Build history of the part. All positions in model axes, mm. Face numbers are marked on the shaded views. Give positions to 0.01 mm unless a question says otherwise; leave off trailing zeros. Order: outer loops, then holes, each group sorted by start corner. A loop starts at its lowest first (then second) coordinate and runs counter-clockwise, first axis right, second up. Notation, with made-up numbers: (43, -1) - (59, -1) arc R23 ccw to (59, 35) - close; hole circle Ø11 at (65.25, 61.25). An arc over 180 degrees is marked (long way). Write each question's results on one line, items separated by ' | '. Start each with the question number.
1) Drop flat-ended pins along their axis: pin 1 Ø2 at (x, y) = (-3.5, -59) entering from +Z; pin 2 Ø3 at (x, y) = (0, 8) entering from -Z; pin 3 Ø2 at (x, z) = (-9.5, 2.5) entering from -Y; pin 4 Ø1.5 at (x, z) = (-7, 3.5) entering from -Y. Give the stop position or say it passes through.
2) Two-plate mould, pull along X, no slides. Class the marked faces 1, 2, 3 and 4: +X half, -X half, draft (parallel to the pull), parting line (faces both ways), or undercut.
3) Cut at B-B on z = 2. List the corners of the cut face in (x, y).
4) Cut at D-D on x = 8. List the corners of the cut face in (y, z), plus the area to 3 significant figures.
5) Cut at A-A on x = 0. List the corners of the cut face in (y, z), plus the area to 3 significant figures.
6) Cut at C-C on y = -8. List the corners of the cut face in (x, z).
7) Drill centre lines: line 1 along X through (y, z) = (0, 4.6); line 2 along Y through (x, z) = (0, 4.5); line 3 along Z through (x, y) = (8.5, -7.5). Where is each one in solid material? Low to high. Write a range as from..to.
from build123d import *

# Parameters (mm, degrees)
ESQUISSE1_R             = 15
ESQUISSE1_R_2           = 1.8
ESQUISSE1_R_3           = 4
BOSS_EXTRU_1_DEPTH      = 7
CONG_1_R                = 1.5
CONG_2_R                = 6
ESQUISSE3_R             = 12
ENL_V_MAT_EXTRU_2_DEPTH = 3.5


with BuildPart() as part:
    # Esquisse1 → Boss.-Extru.1 (new body)
    # profile 1 of 2: a face of its own
    with BuildSketch(Plane.XY):
        with BuildLine():
            ThreePointArc((15, 0), (0, -15), (-15, 0))
            Line((-15, 0), (-15, -80))
            Line((-15, -80), (15, -20))
            Line((15, -20), (15, 0))
        make_face()
    # profile 2 of 2: a face of its own
    with BuildSketch(Plane.XY):
        Circle(ESQUISSE1_R)
        with Locations((-8, 0)):
            Circle(ESQUISSE1_R_2, mode=Mode.SUBTRACT)
        with Locations((0, -8)):
            Circle(ESQUISSE1_R_2, mode=Mode.SUBTRACT)
        with Locations((8, 0)):
            Circle(ESQUISSE1_R_2, mode=Mode.SUBTRACT)
        with Locations((0, 8)):
            Circle(ESQUISSE1_R_2, mode=Mode.SUBTRACT)
        Circle(ESQUISSE1_R_3, mode=Mode.SUBTRACT)
    extrude(amount=BOSS_EXTRU_1_DEPTH)

    # Congé1
    cong_1_edges = [part.edges().sort_by_distance(p)[0] for p in [
        (-15, -80, 3.5),
    ]]
    fillet(cong_1_edges, radius=CONG_1_R)

    # Congé2
    cong_2_edges = [part.edges().sort_by_distance(p)[0] for p in [
        (15, -20, 3.5),
    ]]
    fillet(cong_2_edges, radius=CONG_2_R)

    # Esquisse3 → Enlèv. mat.-Extru.2 (cut)
    with BuildSketch(Plane(origin=(0, 0, 0), x_dir=(-1, 0, 0), z_dir=(0, 0, -1))):
        Circle(ESQUISSE3_R)
    extrude(amount=-ENL_V_MAT_EXTRU_2_DEPTH, mode=Mode.SUBTRACT)


solid = part.part
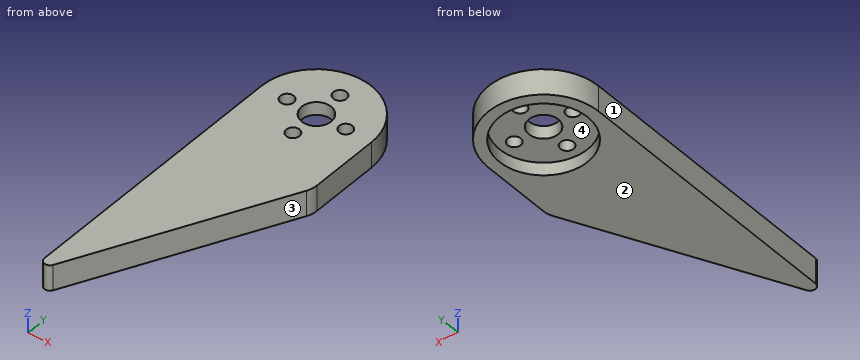
Results:
1) pin 1: z = 7 | pin 2: through | pin 3: y = -71 | pin 4: y = -65.5
2) face 1: -X half | face 2: draft | face 3: +X half | face 4: undercut
3) outline: (-15, -73.65) arc R1.5 ccw to (-12.16, -74.32) - (14.37, -21.27) arc R6 ccw to (15, -18.58) - (15, 0) arc R15 ccw to (-15, 0) - close; hole circle Ø24 at (0, 0)
4) outline: (-34, 0) - (-8.94, 0) - (-8.94, 3.5) - (-1.8, 3.5) - (-1.8, 7) - (-34, 7) - close; (1.8, 3.5) - (8.94, 3.5) - (8.94, 0) - (12.69, 0) - (12.69, 7) - (1.8, 7) - close | area: 252 mm^2
5) outline: (-50, 0) - (-12, 0) - (-12, 3.5) - (-9.8, 3.5) - (-9.8, 7) - (-50, 7) - close; (-6.2, 3.5) - (-4, 3.5) - (-4, 7) - (-6.2, 7) - close; (4, 3.5) - (6.2, 3.5) - (6.2, 7) - (4, 7) - close; (9.8, 3.5) - (12, 3.5) - (12, 0) - (15, 0) - (15, 7) - (9.8, 7) - close | area: 318 mm^2
6) outline: (-15, 0) - (-8.94, 0) - (-8.94, 3.5) - (-1.8, 3.5) - (-1.8, 7) - (-15, 7) - close; (1.8, 3.5) - (8.94, 3.5) - (8.94, 0) - (15, 0) - (15, 7) - (1.8, 7) - close
7) line 1: -15..-9.8, -6.2..-4, 4..6.2, 9.8..15 | line 2: -50..-9.8, -6.2..-4, 4..6.2, 9.8..15 | line 3: 3.5..7
